Input: dimensioned drawing with shaded views. Units: mm. Origin: part minimum x, y, z. A direction names the side the tool comes from. Round coordinates to 2 decimals unless told otherwise and drop trailing zeros. Loops run counter-clockwise (first coordinate to the right, second up) from the corner with the lowest first, then second, coordinate; pieces in that order, holes last. Notation, with made-up numbers: (-22, 80.5) - (22, 80.5) arc R15 ccw to (22, 95.5) - close; hole circle Ø7 at (87.5, 66.25). An arc over 180 degrees is marked (long way). Answer as CSV lines item,"result".
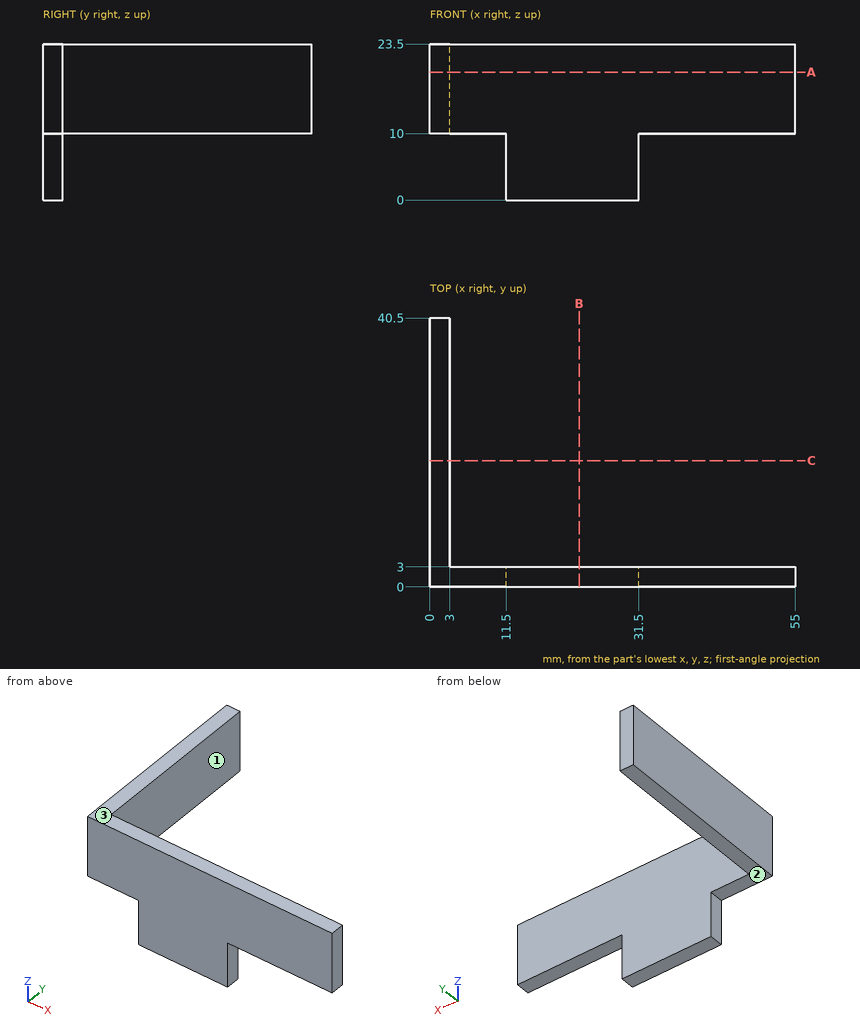
(1) Material intervals for line 1 along Y through (x, z) = (24, 12), sorted ascending.
Findings below:
line 1,"0 to 3"
(2) Section B-B (x = 22.5). Output: boundary loops of the cut face in (y, z).
Findings below:
outline,"(0, 0) - (3, 0) - (3, 23.5) - (0, 23.5) - close"
(3) Section A-A (z = 19.25). Output: boundary loops of the cut face in (x, y), and give its area (4 significant figures).
Findings below:
outline,"(0, 0) - (55, 0) - (55, 3) - (3, 3) - (3, 40.5) - (0, 40.5) - close"
area,"277.5 mm2"
(4) Pin query (flat end, axial travel): P1, Ø3.5, axis at y = 1.5, z = 6.5, coming from the +X side; P2, Ø3, axis at x = 27.5, z = 11, coming from the -Y side; P3, Ø0.9, axis at y = 1.5, z = 6.5, coming from the -X side; P4, Ø3.5, axis at x = 4.5, y = 19.5, coming from the -Z side. Return the tip coordinate at first contact, or that it passes through.
Findings below:
P1,"x = 31.5"
P2,"y = 0"
P3,"x = 11.5"
P4,"z = 10"
(5) Access query for the marked faces 1, 2 and 3. Directions: +Z, -Z, +X, -X, +Y, -Y. A direction counts if a zero-diameter tool reaches every point of the face in a straight line with its end or side. Return the directions, or none.
Findings below:
face 1,"+Z, -Z, +X, +Y"
face 2,"-Z, -X, +Y, -Y"
face 3,"+Z, +X, -X, +Y, -Y"
(6) Section C-C (y = 19). Output: boundary loops of the cut face in (x, z).
Findings below:
outline,"(0, 10) - (3, 10) - (3, 23.5) - (0, 23.5) - close"
